Verification items for the finished model (mm, model axes). A direction names the side the tool comes from. Round coordinates to 2 decimals unless told otherwise and drop trailing zeros. Loops run counter-clockwise (first coordinate to the right, second up) from the corner with the lowest first, then second, coordinate; pieces in that order, holes last.
from build123d import *

# Parameters (mm, degrees)
SKETCH1_W           = 5.461
SKETCH1_H           = 25.4
BOSS_EXTRUDE1_DEPTH = 5.588
CIRPATTERN1_COUNT   = 3
SKETCH3_R           = 3.175
CUT_EXTRUDE1_DEPTH  = 6.588
FILLET2_R           = 6.35


with BuildPart() as part:
    # Sketch1 → Boss-Extrude1 (new body)
    with BuildSketch(Plane(origin=(0, 0, 0), x_dir=(1, 0, 0), z_dir=(0, 1, 0))):
        Polygon((0, 0), (50.8, 29.329393675), (22.225, 152.4), (-22.225, 152.4), (-50.8, 29.329393675), align=None)
        with BuildLine():
            Line((-9.525, 29.329393675), (-9.525, 139.7))
            ThreePointArc((-9.525, 139.7), (-12.7, 142.875), (-15.875, 139.7))
            Line((-15.875, 139.7), (-15.875, 29.329393675))
            ThreePointArc((-15.875, 29.329393675), (-12.7, 26.154393675), (-9.525, 29.329393675))
        make_face(mode=Mode.SUBTRACT)
        with Locations((0, 63.5)):
            Rectangle(SKETCH1_W, SKETCH1_H, mode=Mode.SUBTRACT)
        with BuildLine():
            Line((9.525, 29.329393675), (9.525, 139.7))
            ThreePointArc((9.525, 139.7), (12.7, 142.875), (15.875, 139.7))
            Line((15.875, 139.7), (15.875, 29.329393675))
            ThreePointArc((15.875, 29.329393675), (12.7, 26.154393675), (9.525, 29.329393675))
        make_face(mode=Mode.SUBTRACT)
        with Locations((0, 114.3)):
            Rectangle(SKETCH1_W, SKETCH1_H, mode=Mode.SUBTRACT)
    boss_extrude1 = extrude(amount=BOSS_EXTRUDE1_DEPTH)

    # CirPattern1: Boss-Extrude1 ×3 about axis
    cirpattern1_axis = Axis((0, 0, 0), (0, 1, 0))
    for i in range(1, CIRPATTERN1_COUNT):
        add(boss_extrude1.rotate(cirpattern1_axis, i * 360 / CIRPATTERN1_COUNT))

    # Sketch3 → Cut-Extrude1 (cut, through all)
    with BuildSketch(Plane(origin=(0, 5.588, 0), x_dir=(1, 0, 0), z_dir=(0, 1, 0))):
        Circle(SKETCH3_R)
    extrude(amount=-CUT_EXTRUDE1_DEPTH, mode=Mode.SUBTRACT)

    # Fillet2
    fillet2_edges = [part.edges().sort_by_distance(p)[0] for p in [
        (-143.094771537, 2.794, 56.952585401),
        (-120.869771537, 2.794, 95.447414599),
        (-50.8, 2.794, -29.329393675),
        (-22.225, 2.794, -152.4),
        (22.225, 2.794, -152.4),
        (50.8, 2.794, -29.329393675),
        (0, 2.794, 58.65878735),
        (120.869771537, 2.794, 95.447414599),
        (143.094771537, 2.794, 56.952585401),
    ]]
    fillet(fillet2_edges, radius=FILLET2_R)


solid = part.part
1. Section check C-C (y = 2.3). Give the number of separate pieces and of enclosed holes in the cut face, then the cut area to 3 significant figures.
2. Scan lines: L1, parallel to Z at x = 0, y = 1.45 (3 decimals); L2, parallel to X at y = 4.65, z = -119.5 (1 decimal); L3, parallel to X at y = 2.2, z = -104 (1 decimal). Record each from-to range of solid material in increasing order.
3. Section check B-B (x = -95). Enter the section's corners in (y, z).
4. Release check for a two-part mould opening along Z. For faces 4 (the face through (-95.2, 2.75, 12.18)), 5 (the face through (4, 0, 0)), 6 (the face through (81.798, 2.755, 28.895)) record: released by +Z, released by -Z, zero draft, split by the parting line, or undercut.
5. Tool access check on faces 1 (the face through (-59.746, 2.755, 76.843)), 2 (the face through (4, 5.588, 0)), 3 (the face through (-65.92, 2.75, 56.39)). Record the directions out of +Z, -Z, +X, -X, +Y, -Y that give a thin tool (end or side, any length) a straight path to the whole face; none if there is none.
6. Section check D-D (z = -20). Enter the section's corners in (x, y).
7. Gauge pin test, flat ends, axial feed: P1, Ø1.7, axis at y = 3.5, z = -112.5, coming from the +X side; P2, Ø1.6, axis at x = -1.5, y = 2, coming from the +Z side; P3, Ø1.7, axis at y = 3.5, z = -64.5, coming from the +X side. Record the tip position at first contact, or that the pin passes through.
8. Section check A-A (x = -12.7). Enter the section's corners in (y, z) (3 decimals), then the cut area to 3 significant figures.
Taken from the geometry:
1. separate pieces: 1
1. enclosed holes: 13
1. area: 26,100 mm2
2. L1: z = -152.4 to -127, -101.6 to -76.2, -50.8 to -3.175, 3.175 to 58.946
2. L2: x = -29.9 to -15.9, -9.5 to -2.7, 2.7 to 9.5, 15.9 to 29.9
2. L3: x = -33.5 to -15.9, -9.5 to -2.7, 2.7 to 9.5, 15.9 to 33.5
3. outline: (0, 11.99) - (5.59, 11.99) - (5.59, 36.52) - (0, 36.52) - close; (0, 43.85) - (5.59, 43.85) - (5.59, 51.7) - (0, 51.7) - close; (0, 58) - (5.59, 58) - (5.59, 65.85) - (0, 65.85) - close; (0, 73.18) - (5.59, 73.18) - (5.59, 87.57) - (0, 87.57) - close
4. face 4: released by -Z
4. face 5: zero draft
4. face 6: undercut
5. face 1: +Z, +Y, -Y
5. face 2: +Z, -Z, +X, -X, +Y
5. face 3: +Y, -Y
6. outline: (-60.78, 0) - (60.78, 0) - (60.78, 5.59) - (-60.78, 5.59) - close
7. P1: stops at x = 31.69
7. P2: stops at z = 59.36
7. P3: stops at x = 42.83
8. outline: (0, -152.4) - (5.588, -152.4) - (5.588, -142.875) - (0, -142.875) - close; (0, -26.154) - (5.588, -26.154) - (5.588, 62.524) - (0, 62.524) - close
8. area: 549 mm2
